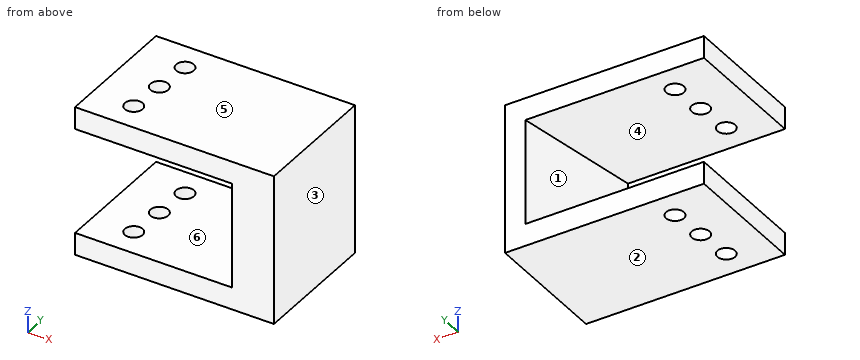
```python
from build123d import *

# Parameters (mm, degrees)
SALIENTE_EXTRUIR1_DEPTH   = 2
SALIENTE_EXTRUIR2_DEPTH   = 11.5
CROQUIS3_W                = 17.909938215
CROQUIS3_H                = 11.583193085
SALIENTE_EXTRUIR3_DEPTH   = 2
TALADRO_ROSCADO_M21_D     = 1.6
TALADRO_ROSCADO_M21_DEPTH = 17
TALADRO_ROSCADO_M21_TIP   = 0.480688495


with BuildPart() as part:
    # Croquis1 → Saliente-Extruir1 (new body)
    with BuildSketch(Plane.XY.offset(-8.1)):
        Polygon((-4.56285844, -53.408133883), (-6.500165269, -64.991326968), (-20.63641004, -64.991326968), (-20.63641004, -53.408133883), align=None)
    extrude(amount=SALIENTE_EXTRUIR1_DEPTH)

    # Croquis2 → Saliente-Extruir2 (add)
    with BuildSketch(Plane.XY.offset(-6.1)):
        Polygon((-4.56285844, -53.408133883), (-2.726471825, -53.408133883), (-2.726471825, -64.991326968), (-6.500165269, -64.991326968), align=None)
    extrude(amount=-SALIENTE_EXTRUIR2_DEPTH)

    # Croquis3 → Saliente-Extruir3 (add)
    with BuildSketch(Plane(origin=(0, 0, -17.6), x_dir=(-1, 0, 0), z_dir=(0, 0, -1))):
        with Locations((11.681440933, -59.199730426)):
            Rectangle(CROQUIS3_W, CROQUIS3_H)
    extrude(amount=SALIENTE_EXTRUIR3_DEPTH)

    # Taladro roscado M21
    with Locations(Plane.XY.offset(-6.1)):
        with Locations((-16.926929895, -62.491326968), (-16.691574413, -59.199730426), (-16.456218931, -55.908133883)):
            Hole(TALADRO_ROSCADO_M21_D / 2, depth=TALADRO_ROSCADO_M21_DEPTH)
            with Locations((0, 0, -(TALADRO_ROSCADO_M21_DEPTH + TALADRO_ROSCADO_M21_TIP / 2))):  # 118° drill point
                Cone(0, TALADRO_ROSCADO_M21_D / 2, TALADRO_ROSCADO_M21_TIP, mode=Mode.SUBTRACT)


solid = part.part
```
Source: CAD feature listing. Evaluate the final solid. Frame: model axes, mm. Face numbers are marked on the shaded views. A direction names the side the tool comes from. Coordinates: 2 decimals unless noted, no trailing zeros. Write each loop counter-clockwise with the first axis right and the second up, starting at its lowest first coordinate (ties: lowest second). Pieces come first, ordered by that corner, then holes. Notation, with made-up numbers: (-8, 78.5) -> (43, 78.5) arc R27 ccw to (43, 99.5) -> close; hole circle Ø8 at (-32.5, 88). An arc over 180 degrees is marked (long way). Return JSON: item names as keys, results as strings. Group by question number.
1) Ray query, line 1 along Z through (x, y) = (-11.5, -59.5); line 2 along X through (y, z) = (-56.25, -15); line 3 along X through (y, z) = (-58, -14.75). Return the intervals inside material, ascending.
2) Set-up query: the marked faces 1 and 2. Return all of +Z, -Z, +X, -X, +Y, -Y with unobstructed straight access to the full face (end or side cutting, diameter ignored); none if empty.
3) Section query D-D, the plane x = -5.25. Return loops of the section in (y, z).
4) Section query B-B, the plane y = -56.25. Return loops of the section in (x, z).
5) Mould query, pull axis Z, two halves, no side actions, for the marked faces 3, 4, 5 and 6. Classes: +Z half, -Z half, draft (parallel to the pull), parting line (faces both ways), or undercut.
6) Section query C-C, the plane z = -15.5. Return loops of the section in (x, y), plus the area to 3 significant figures.
7) Contact query for flat-ended pins moving along their axis: P1, Ø1, axis at x = -9.5, z = -8.5, coming from the +Y side; P2, Ø2, axis at y = -60, z = -15, coming from the -X side. Output: stop coordinate, or through.
8) Section query A-A, the plane x = -9. Return loops of the section in (y, z).
From the geometry:
{
 "1": {"line 1": "-19.6 to -17.6, -8.1 to -6.1", "line 2": "-5.04 to -2.73", "line 3": "-5.33 to -2.73"},
 "2": {"face 1": "-X, +Y", "face 2": "-Z, +X, -X, +Y, -Y"},
 "3": {"outline": "(-64.99, -19.6) -> (-53.41, -19.6) -> (-53.41, -17.6) -> (-57.52, -17.6) -> (-57.52, -8.1) -> (-53.41, -8.1) -> (-53.41, -6.1) -> (-64.99, -6.1) -> close"},
 "4": {"outline": "(-20.64, -19.6) -> (-17.18, -19.6) -> (-17.18, -17.6) -> (-20.64, -17.6) -> close; (-20.64, -8.1) -> (-17.18, -8.1) -> (-17.18, -6.1) -> (-20.64, -6.1) -> close; (-15.73, -19.6) -> (-2.73, -19.6) -> (-2.73, -6.1) -> (-15.73, -6.1) -> (-15.73, -8.1) -> (-5.04, -8.1) -> (-5.04, -17.6) -> (-15.73, -17.6) -> close"},
 "5": {"face 3": "draft", "face 4": "undercut", "face 5": "+Z half", "face 6": "undercut"},
 "6": {"outline": "(-6.5, -64.99) -> (-2.73, -64.99) -> (-2.73, -53.41) -> (-4.56, -53.41) -> close", "area": "32.5 mm²"},
 "7": {"P1": "y = -53.41", "P2": "x = -5.83"},
 "8": {"outline": "(-64.99, -19.6) -> (-53.41, -19.6) -> (-53.41, -17.6) -> (-64.99, -17.6) -> close; (-64.99, -8.1) -> (-53.41, -8.1) -> (-53.41, -6.1) -> (-64.99, -6.1) -> close"}
}
